Work out the finished part from the listing and answer in its coordinate system (mm). A direction names the side the tool comes from. Coordinates: 2 decimals unless noted, no trailing zeros. Order: outer loops, then holes, each group sorted by start corner. A loop starts at its lowest first (then second) coordinate and runs counter-clockwise, first axis right, second up. Notation, with made-up numbers: (14, -21.5) -> (32, -21.5) arc R10 ccw to (32, -17.5) -> close; hole circle Ø2 at (-12.75, 70.25). An arc over 180 degrees is marked (long way). Use one line per item in the form item = value.
from build123d import *

# Parameters (mm, degrees)
SKETCH1_W                    = 60
SKETCH1_H                    = 50
BASE_FLANGE1_DEPTH           = 3
EDGE_FLANGE1_STRIP_W         = 18
EDGE_FLANGE1_STRIP_H         = 3
EDGE_FLANGE1_STRIP_CUT_DEPTH = 50
EDGE_FLANGE1_DEPTH           = 50
CUT_EXTRUDE1_DEPTH           = 10
SKETCH10_R                   = 3.5
SKETCH10_R_2                 = 1.665
CUT_EXTRUDE2_DEPTH           = 10


# Sheet-metal steps are written as plain solids
with BuildPart() as part:
    # Sketch1 → Base-Flange1 (new body)
    with BuildSketch(Plane.XY):
        Rectangle(SKETCH1_W, SKETCH1_H)
    extrude(amount=-BASE_FLANGE1_DEPTH)

    # Edge-Flange1 strip (across the edge) → Edge-Flange1 strip cut (cut)
    with BuildSketch(Plane(origin=(30, -25, 0), x_dir=(-1, 0, 0), z_dir=(0, 1, 0))):
        with Locations((-3, -1.5)):
            Rectangle(EDGE_FLANGE1_STRIP_W, EDGE_FLANGE1_STRIP_H)
    extrude(amount=EDGE_FLANGE1_STRIP_CUT_DEPTH, mode=Mode.SUBTRACT)

    # Edge-Flange1 section (across the edge) → Edge-Flange1 (add)
    with BuildSketch(Plane(origin=(30, -25, 0), x_dir=(-1, 0, 0), z_dir=(0, 1, 0))):
        with BuildLine():
            Line((0, 3), (0, 57))
            Line((0, 57), (3, 57))
            Line((3, 57), (3, 3))
            ThreePointArc((3, 3), (3.878679656, 0.878679656), (6, 0))
            Line((6, 0), (6, -3))
            ThreePointArc((6, -3), (1.757359313, -1.242640687), (0, 3))
        make_face()
    extrude(amount=EDGE_FLANGE1_DEPTH)

    # Sketch9 → Cut-Extrude1 (cut)
    with BuildSketch(Plane(origin=(30, 0, 0), x_dir=(0, 0, -1), z_dir=(1, 0, 0))):
        with BuildLine():
            Line((-30, 25), (-57, 25))
            Line((-57, 25), (-57, -25))
            Line((-57, -25), (-30, -25))
            ThreePointArc((-30, -25), (-55, 0), (-30, 25))
        make_face()
    extrude(amount=-CUT_EXTRUDE1_DEPTH, mode=Mode.SUBTRACT)

    # Sketch10 → Cut-Extrude2 (cut)
    with BuildSketch(Plane(origin=(30, 0, 0), x_dir=(0, 0, -1), z_dir=(1, 0, 0))):
        with Locations((-30, 0)):
            Circle(SKETCH10_R)
        with Locations((-30, 12.5)):
            Circle(SKETCH10_R_2)
        with Locations((-42.5, 0)):
            Circle(SKETCH10_R_2)
        with Locations(Location((-30, -12.5, 0), (0, 0, 180))):
            Circle(SKETCH10_R_2)
        with Locations(Location((-17.5, 0, 0), (0, 0, 180))):
            Circle(SKETCH10_R_2)
    extrude(amount=-CUT_EXTRUDE2_DEPTH, mode=Mode.SUBTRACT)


solid = part.part
(1) Section C-C on y = -17.5 is taken. Write down the section's boundary in (x, z).
Data:
outline = (-30, -3) -> (24, -3) arc R6 ccw to (30, 3) -> (30, 47.85) -> (27, 47.85) -> (27, 3) arc R3 cw to (24, 0) -> (-30, 0) -> close
(2) Each of these flat-tipped pins is pushed along its axis until it touches: P1, Ø3, axis at y = 4, z = 9, coming from the -X side; P2, Ø10, axis at x = -22.5, y = 6.5, coming from the +Z side. Where does it stop, or does it pass through?
Data:
P1 = 27
P2 = 0
(3) Section D-D on z = 7 is taken. Write down the section's boundary in (x, y), plus the area to 3 significant figures.
Data:
outline = (27, -25) -> (30, -25) -> (30, 25) -> (27, 25) -> close
area = 150 mm²
(4) Section A-A on y = 0 is taken. Write down the section's boundary in (x, z) (3 decimals), plus the area to 3 significant figures.
Data:
outline = (-30, -3) -> (24, -3) arc R6 ccw to (30, 3) -> (30, 15.835) -> (27, 15.835) -> (27, 3) arc R3 cw to (24, 0) -> (-30, 0) -> close; (27, 19.165) -> (30, 19.165) -> (30, 26.5) -> (27, 26.5) -> close; (27, 33.5) -> (30, 33.5) -> (30, 40.835) -> (27, 40.835) -> close; (27, 44.165) -> (30, 44.165) -> (30, 55) -> (27, 55) -> close
area = 298 mm²
(5) Straight lines are drawn through the part: line 1 along Y through (x, z) = (28.7, 30) (3 decimals); line 2 along Y through (x, z) = (27.8, 17.5) (3 decimals); line 3 along Z through (x, y) = (12, 2.5). For each, find the intervals that lie inside material, in ascending order.
Data:
line_1 = -25 to -14.165, -10.835 to -3.5, 3.5 to 10.835, 14.165 to 25
line_2 = -25 to -1.665, 1.665 to 25
line_3 = -3 to 0
(6) Which of the six approach directions +Z, -Z, +X, -X, +Y, -Y give full straight-line access (tool end or side, diameter ignored) to faces 1 (the flat face through (27, 0, 24)), 2 (the cylindrical face through (28.521, -0.073, 15.837))?
Data:
face_1 = +Z, -X, +Y, -Y
face_2 = +X, -X
(7) Section B-B on z = 17.5 is taken. Write down the section's boundary in (x, y) (3 decimals), plus the area to 3 significant figures.
Data:
outline = (27, -25) -> (30, -25) -> (30, -1.665) -> (27, -1.665) -> close; (27, 1.665) -> (30, 1.665) -> (30, 25) -> (27, 25) -> close
area = 140 mm²
(8) The mould has two halves that part along Z. Classify faces 3 (the cylindrical face through (26.14, -0.35, 0.9)), 4 (the cylindrical face through (28.521, 12.573, 31.663)), 5 (the flat face through (9, 25, -1)), 6 (the cylindrical face through (28.196, -0.35, -1.289)): released by +Z, released by -Z, zero draft, split by the parting line, or undercut.
Data:
face_3 = released by +Z
face_4 = undercut
face_5 = zero draft
face_6 = released by -Z
